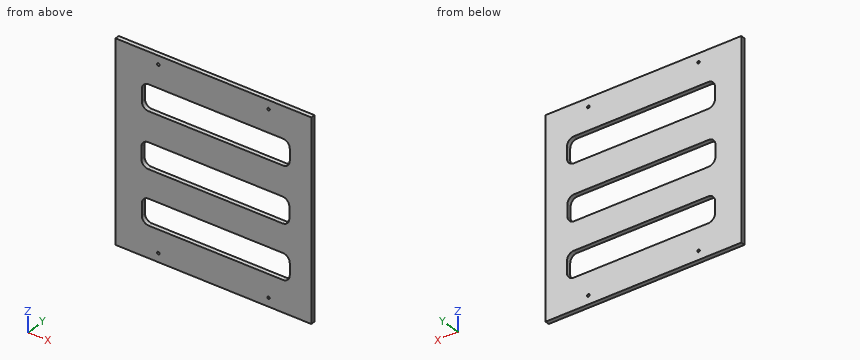
```python
from build123d import *

# Parameters (mm, degrees)
SKETCH1_W           = 229
SKETCH1_H           = 229
SKETCH1_R           = 1.5
BOSS_EXTRUDE1_DEPTH = 5
CUT_EXTRUDE1_DEPTH  = 5


with BuildPart() as part:
    # Sketch1 → Boss-Extrude1 (new body)
    with BuildSketch(Plane(origin=(0, 0, 0), x_dir=(1, 0, 0), z_dir=(0, 1, 0))):
        with Locations((114.5, -114.5)):
            Rectangle(SKETCH1_W, SKETCH1_H)
        with Locations(Location((179, -10, 0), (0, 0, 270))):
            Circle(SKETCH1_R, mode=Mode.SUBTRACT)
        with Locations(Location((50, -10, 0), (0, 0, 90))):
            Circle(SKETCH1_R, mode=Mode.SUBTRACT)
        with Locations(Location((179, -219, 0), (0, 0, 90))):
            Circle(SKETCH1_R, mode=Mode.SUBTRACT)
        with Locations(Location((50, -219, 0), (0, 0, 270))):
            Circle(SKETCH1_R, mode=Mode.SUBTRACT)
    extrude(amount=BOSS_EXTRUDE1_DEPTH)

    # Sketch2 → Cut-Extrude1 (cut)
    with BuildSketch(Plane(origin=(0, 5, 0), x_dir=(1, 0, 0), z_dir=(0, 1, 0))):
        with BuildLine():
            Line((38.760316137, -36.197957946), (195.832686867, -36.197957946))
            ThreePointArc((195.832686867, -36.197957946), (201.489541116, -38.541103697), (203.832686867, -44.197957946))
            Line((203.832686867, -44.197957946), (203.832686867, -58.0273073))
            ThreePointArc((203.832686867, -58.0273073), (201.489541116, -63.68416155), (195.832686867, -66.0273073))
            Line((195.832686867, -66.0273073), (38.760316137, -66.0273073))
            ThreePointArc((38.760316137, -66.0273073), (33.103461887, -63.68416155), (30.760316137, -58.0273073))
            Line((30.760316137, -58.0273073), (30.760316137, -44.197957946))
            ThreePointArc((30.760316137, -44.197957946), (33.103461887, -38.541103697), (38.760316137, -36.197957946))
        make_face()
        with BuildLine():
            Line((203.832686867, -184.802042054), (203.832686867, -170.9726927))
            ThreePointArc((203.832686867, -170.9726927), (201.489541116, -165.31583845), (195.832686867, -162.9726927))
            Line((195.832686867, -162.9726927), (38.760316137, -162.9726927))
            ThreePointArc((38.760316137, -162.9726927), (33.103461887, -165.31583845), (30.760316137, -170.9726927))
            Line((30.760316137, -170.9726927), (30.760316137, -184.802042054))
            ThreePointArc((30.760316137, -184.802042054), (33.103461887, -190.458896303), (38.760316137, -192.802042054))
            Line((38.760316137, -192.802042054), (195.832686867, -192.802042054))
            ThreePointArc((195.832686867, -192.802042054), (201.489541116, -190.458896303), (203.832686867, -184.802042054))
        make_face()
        with BuildLine():
            Line((38.22, -98.653158156), (195.29, -98.653158156))
            ThreePointArc((195.29, -98.653158156), (200.946854249, -100.996303906), (203.29, -106.653158156))
            Line((203.29, -106.653158156), (203.29, -120.48250751))
            ThreePointArc((203.29, -120.48250751), (200.946854249, -126.139361759), (195.29, -128.48250751))
            Line((195.29, -128.48250751), (38.22, -128.48250751))
            ThreePointArc((38.22, -128.48250751), (32.563145751, -126.139361759), (30.22, -120.48250751))
            Line((30.22, -120.48250751), (30.22, -106.653158156))
            ThreePointArc((30.22, -106.653158156), (32.563145751, -100.996303906), (38.22, -98.653158156))
        make_face()
    extrude(amount=-CUT_EXTRUDE1_DEPTH, mode=Mode.SUBTRACT)


solid = part.part
```
Could you check a few things on this model? Use its own coordinates, in mm. Coordinates: 2 decimals unless noted, no trailing zeros. Order: outer loops, then holes, each group sorted by start corner. A loop starts at its lowest first (then second) coordinate and runs counter-clockwise, first axis right, second up. Notation, with made-up numbers: M 77.25,72 L 108.25,72 A14 cw 108.25,87 Z; hole C 35,63.5 d7. An arc over 180 degrees is marked long. Use one line per item in the form item = value. Start each with the question number.
1. Suppose I cut it at A-A on x = 58. Write out the boundary of the cut face in (y, z), then the cut area to 3 significant figures.
2. Please list where these lines run through material, in increasing order: line 1 (Z direction, x = 170, y = 1.25); line 2 (Z direction, x = 179, y = 2.9); line 3 (X direction, y = 2.6, z = 10).
3. Suppose I cut it at B-B on y = 2.2. Count the separate pieces of the cut face and the enclosed holes in it, then the cut area to 3 significant figures.
4. Suppose I cut it at C-C on z = 124.5. Write out the boundary of the cut face in (x, y).
5. For pin 1 (3.5 mm diameter, centred on x = 50, z = 219, fed in from -Y), with a flat end and sliding along its axis, tell me the tip position at first contact or that it passes through.
Geometry says:
q1.outline = M 0,0 L 5,0 L 5,36.2 L 0,36.2 Z; M 0,66.03 L 5,66.03 L 5,98.65 L 0,98.65 Z; M 0,128.48 L 5,128.48 L 5,162.97 L 0,162.97 Z; M 0,192.8 L 5,192.8 L 5,229 L 0,229 Z
q1.area = 698 mm^2
q2.line_1 = 0 to 36.2, 66.03 to 98.65, 128.48 to 162.97, 192.8 to 229
q2.line_2 = 0 to 8.5, 11.5 to 36.2, 66.03 to 98.65, 128.48 to 162.97, 192.8 to 217.5, 220.5 to 229
q2.line_3 = 0 to 48.5, 51.5 to 177.5, 180.5 to 229
q3.separate_pieces = 1
q3.enclosed_holes = 7
q3.area = 37,100 mm^2
q4.outline = M 0,0 L 31.3,0 L 31.3,5 L 0,5 Z; M 202.21,0 L 229,0 L 229,5 L 202.21,5 Z
q5.pin_1 = 0
